from build123d import *

# Parameters (mm, degrees)
ESQUISSE1_W             = 130
ESQUISSE1_H             = 50
BOSS_EXTRU_1_DEPTH      = 100
ESQUISSE2_W             = 44
ESQUISSE2_H             = 40
ENL_V_MAT_EXTRU_1_DEPTH = 127
ESQUISSE3_W             = 44
ESQUISSE3_H             = 40
ENL_V_MAT_EXTRU_2_DEPTH = 127
COQUE1_START            = -47
COQUE1_OUTLINE_W        = 127
COQUE1_OUTLINE_H        = 8
COQUE1_DEPTH            = 44


# Read off the part's stored shape, not the designer's step: Coque1
with BuildPart() as part:
    # Esquisse1 → Boss.-Extru.1 (new body)
    with BuildSketch(Plane(origin=(0, 0, 0), x_dir=(1, 0, 0), z_dir=(0, 1, 0))):
        with Locations((65, 25)):
            Rectangle(ESQUISSE1_W, ESQUISSE1_H)
    extrude(amount=BOSS_EXTRU_1_DEPTH)

    # Esquisse2 → Enlèv. mat.-Extru.1 (cut)
    with BuildSketch(Plane(origin=(130, 0, 0), x_dir=(0, 0, -1), z_dir=(1, 0, 0))):
        with Locations((25, 77)):
            Rectangle(ESQUISSE2_W, ESQUISSE2_H)
    extrude(amount=-ENL_V_MAT_EXTRU_1_DEPTH, mode=Mode.SUBTRACT)

    # Esquisse3 → Enlèv. mat.-Extru.2 (cut)
    with BuildSketch(Plane(origin=(130, 0, 0), x_dir=(0, 0, -1), z_dir=(1, 0, 0))):
        with Locations((25, 34)):
            Rectangle(ESQUISSE3_W, ESQUISSE3_H)
    extrude(amount=-ENL_V_MAT_EXTRU_2_DEPTH, mode=Mode.SUBTRACT)

    # Coque1 outline → Coque1 (cut)
    with BuildSketch(Plane.XY.offset(COQUE1_START)):
        with Locations((66.5, 7)):
            Rectangle(COQUE1_OUTLINE_W, COQUE1_OUTLINE_H)
    extrude(amount=COQUE1_DEPTH, mode=Mode.SUBTRACT)


solid = part.part
For this review, take the finished solid that the model builds, in its own axes (mm). A direction names the side the tool comes from. Round coordinates to 2 decimals unless told otherwise and drop trailing zeros. Loops run counter-clockwise (first coordinate to the right, second up) from the corner with the lowest first, then second, coordinate; pieces in that order, holes last. Notation, with made-up numbers: (-5.5, 32.5) - (41.5, 32.5) arc R14 cw to (41.5, 47.5) - close; hole circle Ø10 at (-21.5, 77). An arc over 180 degrees is marked (long way). One line per question, with ' | ' between items.
Q1. The part is to be moulded in two halves that separate along Z. For faces 1 (the flat face through (67, 77, -47)), 2 (the flat face through (64, 100, -25)), 3 (the flat face through (64, 49, -50)), say which applies: released by +Z, released by -Z, zero draft, split by the parting line, or undercut.
Taken from the geometry:
face 1: undercut | face 2: zero draft | face 3: released by -Z
Q2. Take a section at B-B (z = -38.5). Give the boundary of the cut face in (x, y).
Taken from the geometry:
outline: (0, 0) - (130, 0) - (130, 3) - (3, 3) - (3, 11) - (130, 11) - (130, 14) - (3, 14) - (3, 54) - (130, 54) - (130, 57) - (3, 57) - (3, 97) - (130, 97) - (130, 100) - (0, 100) - close
Q3. Tool access review of faces 4 (the flat face through (67, 54, -25)), 5 (the flat face through (64, 0, -25)): name each direction out of +Z, -Z, +X, -X, +Y, -Y from which nothing blocks a thin tool from reaching the whole face with its end or side.
Taken from the geometry:
face 4: +X | face 5: +Z, -Z, +X, -X, -Y
Q4. Take a section at A-A (x = 102). Give the boundary of the cut face in (y, z), and give its area (3 significant figures).
Taken from the geometry:
outline: (0, -50) - (100, -50) - (100, 0) - (0, 0) - close; hole (3, -47) - (11, -47) - (11, -3) - (3, -3) - close; hole (14, -47) - (54, -47) - (54, -3) - (14, -3) - close; hole (57, -47) - (97, -47) - (97, -3) - (57, -3) - close | area: 1,130 mm²
Q5. For pin 1 (12 mm diameter, centred on y = 27.5, z = -27, fed in from +X), flat-tipped, find the tip position at first contact; note if it passes through.
Taken from the geometry:
pin 1: stops at x = 3
Q6. For line 1 along Y through (x, z) = (98, -40); line 2 along Z through (x, y) = (41, 86); line 3 along X through (y, z) = (44, -24.5), list the stretches that pass through material, from the lowest coordinate up. Write a range as [from, to].
Taken from the geometry:
line 1: y = [0, 3], [11, 14], [54, 57], [97, 100] | line 2: z = [-50, -47], [-3, 0] | line 3: x = [0, 3]
Q7. Take a section at C-C (y = 47.5). Give the boundary of the cut face in (x, z), and give its area (3 significant figures).
Taken from the geometry:
outline: (0, -50) - (130, -50) - (130, -47) - (3, -47) - (3, -3) - (130, -3) - (130, 0) - (0, 0) - close | area: 912 mm²
